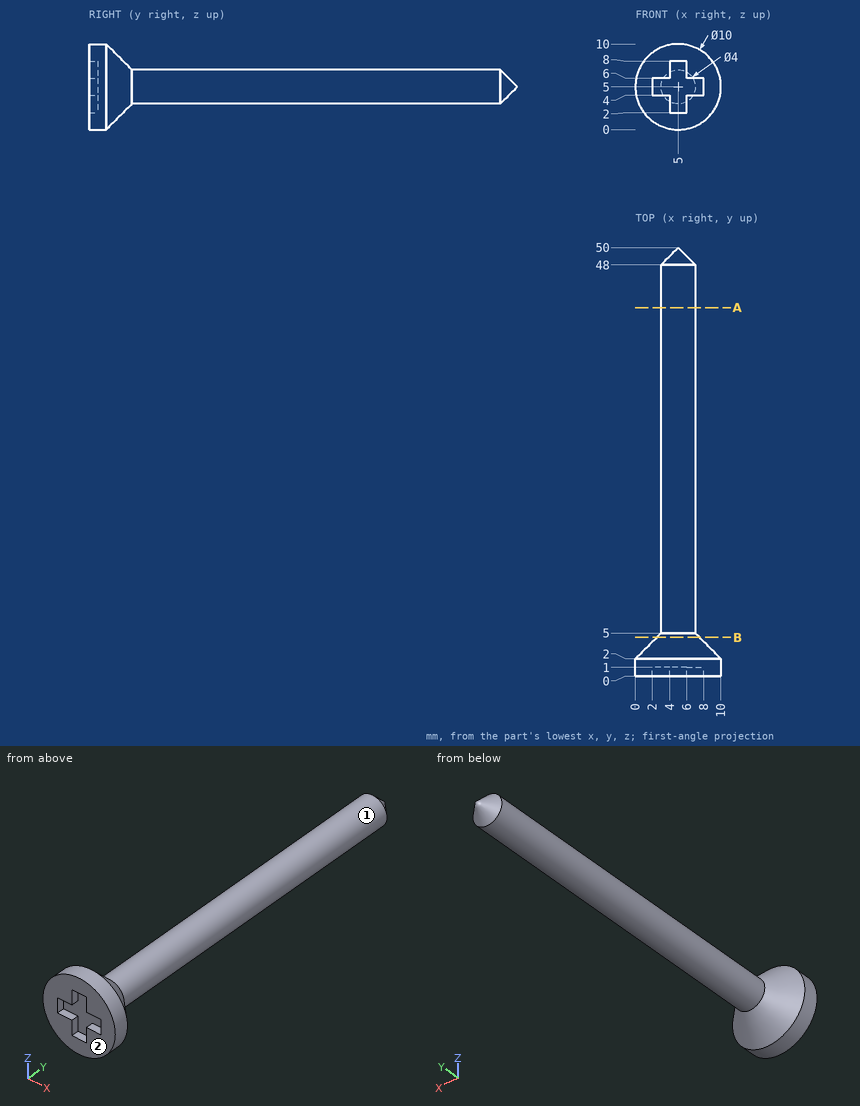
Can you work these out from the drawing? Everything is in mm from the part's minimum corner. A direction names the side the tool comes from. Round coordinates to 2 decimals unless told otherwise and drop trailing zeros. Loops run counter-clockwise (first coordinate to the right, second up) from the corner with the lowest first, then second, coordinate; pieces in that order, holes last. Notation, with made-up numbers: (6.5, 21) -> (25.5, 21) arc R22 cw to (25.5, 55) -> close; hole circle Ø7 at (-39, 81). An arc over 180 degrees is marked (long way). One line per question, with ' | ' between items.
(1) If I drill on probe 1 along X at (y, z) = (30.5, 5); probe 2 along Y at (x, z) = (5.75, 9.75); probe 3 along Y at (x, z) = (4.5, 4.5), over which ranges is the centre line in solid material (lowest first)?
Model answer:
probe 1: x = 3 to 7 | probe 2: y = 0 to 2.19 | probe 3: y = 1 to 49.29
(2) If we section it at A-A on y = 43: List the corners of the cut face in (x, z) for me, and give its area (3 significant figures).
Model answer:
outline: circle Ø4 at (5, 5) | area: 12.6 mm^2
(3) For the marked faces 1 and 2, which set-ups out of +Z, -Z, +X, -X, +Y, -Y let a thin tool reach every point of the face, with its end or its side?
Model answer:
face 1: +Y | face 2: +Z, -Z, +X, -X, -Y
(4) For pin 1 Ø0.5 at (y, z) = (0.5, 3) entering from +X; pin 2 Ø1 at (x, z) = (5.5, 8) entering from +Y; pin 3 Ø0.8 at (x, y) = (7, 0.5) entering from -Z, each with a flat end and sliding along its axis, tell me the tip position at first contact or that it passes through.
Model answer:
pin 1: stops at x = 9.68 | pin 2: stops at y = 4.46 | pin 3: stops at z = 0.26
(5) If we section it at B-B on y = 4.5: List the corners of the cut face in (x, z) for me.
Model answer:
outline: circle Ø5 at (5, 5)
